Could you check a few things on this model? Use its own coordinates, in mm. Face numbers are marked on the shaded views. A direction names the side the tool comes from. Give positions to 0.01 mm unless a question says otherwise; leave off trailing zeros. Write each loop counter-clockwise with the first axis right and the second up, starting at its lowest first coordinate (ties: lowest second). Pieces come first, ordered by that corner, then holes. Notation, with made-up numbers: (-9.5, -5.75) -> (37.5, -5.75) arc R11 ccw to (37.5, 3.25) -> close; hole circle Ø8 at (74, 76.5). An arc over 180 degrees is marked (long way). Write item = value, one per line. Start each with the question number.
Autodesk Inventor part; units mm, degrees
ref_plane "XZ Plane" through (0, 0, 0) normal (0, 1, 0) x (-1, 0, 0)
ref_plane "XY Plane" through (0, 0, 0) normal (0, 0, 1) x (1, 0, 0)
sketch "Skizze1" plane through (0, 0, 0) normal (1, 0, 0) x (0, 1, 0)
  line L0 (15, -20) -> (5, -20)
  line L1 (5, -20) -> (5, -25)
  line L2 (5, -25) -> (15, -25)
  line L3 (15, -25) -> (15, -20)
  line L4 (5, -20) -> (0, -20)
  line L5 (0, -20) -> (0, -55)
  line L6 (0, -55) -> (5, -55)
  line L7 (5, -55) -> (5, -20)
  line L8 (0, -47) -> (-15, -47)
  line L9 (-15, -47) -> (-15, -42)
  line L10 (-15, -42) -> (0, -42)
  line L11 (0, -42) -> (0, -47)
  line L12 (0, -42) -> (-2, -42)
  line L13 (-2, -42) -> (-2, -37.5)
  line L14 (-2, -37.5) -> (0, -37.5)
  line L15 (0, -37.5) -> (0, -42)
  line L16 (-21, 0) -> (21, 0)
  line L17 (0, -66) -> (0, 11)
  point P0 (0, 0)
  point P1 (10, -25)
  point P2 (10, -20)
  point P3 (0, -44.5)
  point P4 (2.5, -55)
  point P5 (-7.5, -47)
  point P6 (0, -37.5)
  point P7 (-2, -42)
  point P8 (5, -25)
  dimension "d0" = 5
  dimension "d1" = 5
  dimension "d2" = 35
  dimension "d3" = 10
  dimension "d4" = 8
  dimension "d5" = 5
  dimension "d6" = 15
  dimension "d7" = 20
  dimension "d8" = 2
  dimension "d9" = 4.5
  dimension "d10" = 0
revolve "Umdrehung1" add sketch "Skizze1" angle 360 about axis through (0, -10, 0) along (0, 1, 0)
fillet "Rundung1" radius 3 1 edges at (0, 5, 25)
fillet "Rundung2" radius 2 1 edges at (0, -2, 42)
sketch "Skizze2" plane through (0, 5, 0) normal (0, 1, 0) x (1, 0, 0)
  line L0 (-77, 0) -> (77, 0)
  line L1 (0, 77) -> (0, -77)
  circle A0 centre (0, 0) radius 51
  circle A1 centre (0, 0) radius 55
  point P0 (0, -51)
  point P1 (44.1673, -25.5)
  point P2 (44.1673, 25.5)
  point P3 (0, 51)
  point P4 (-44.1673, 25.5)
  point P5 (-44.1673, -25.5)
  dimension "d14" = 4
  dimension "d17" = 360
hole "Bohrung1" at (0, 5, 51) at (44.1673, 5, 25.5) at (44.1673, 5, -25.5) at (0, 5, -51) at (-44.1673, 5, -25.5) at (-44.1673, 5, 25.5) direction (0, -1, 0) diameter 4.5 depth 11.8 tip angle 118
properties part number "Deckel Stempel"
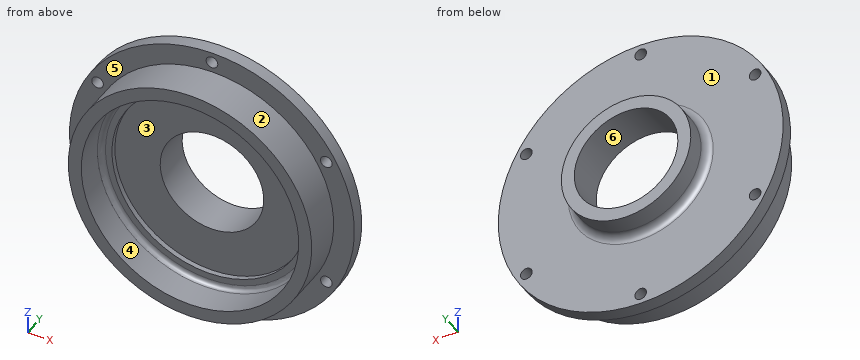
(1) Imagine slicing it at C-C (y = -13). Please give me the cut outline in (x, z), then the cut area to 3 significant figures.
(2) Imagine slicing it at D-D (z = 45.5). Please give me the cut outline in (x, y).
(3) We'd pull the mould along X, two halves only. Please class the marked faces 1, 2, 3 and 4: released by +X, released by -X, zero draft, split by the parting line, or undercut.
(4) On a 3-axis mill with a long thin cutter (end or side, diameter ignored), from which of +Z, -Z, +X, -X, +Y, -Y can I reach the whole of each face in a straight line? I mean the marked faces 5 and 6. Say none if no direction works.
(5) Imagine slicing it at A-A (z = 0). Please give me the cut outline in (x, y), then the cut area to 3 significant figures.
(6) If I drill on line 1 along X through (y, z) = (2.8, 25.5); line 2 along Z through (x, y) = (0, 11.75); line 3 along Y through (x, z) = (45, -30.5), over which ranges is the centre line in solid material (lowest first)? Write a range as from..to.
(7) Imagine slicing it at B-B (x = 0). State how many separate pieces and enclosed holes the cut face has, then the cut area to 3 significant figures.
(8) I'm going to push flat-ended pins straight in: pin 1 (2.5 mm diameter, centred on x = 0, z = -51, fed in from +Y); pin 2 (5 mm diameter, centred on x = 37, z = -6.5, fed in from -Y); pin 3 (6 mm diameter, centred on x = 24.5, z = 20.5, fed in from -Y); pin 4 (2 mm diameter, centred on x = -37, y = 3, fed in from -Z). Where does each tip first touch, or does it pass through?
Answers below:
q1.outline = circle Ø94 at (0, 0); hole circle Ø84 at (0, 0)
q1.area = 1,400 mm^2
q2.outline = (-30.9, 0) -> (-11.78, 0) -> (-11.78, -15) -> (11.78, -15) -> (11.78, 0) -> (30.9, 0) -> (30.9, 5) -> (-30.9, 5) -> close
q3.face_1 = zero draft
q3.face_2 = split by the parting line
q3.face_3 = undercut
q3.face_4 = undercut
q4.face_5 = -Y
q4.face_6 = +Y, -Y
q5.outline = (-55, 0) -> (-47, 0) -> (-47, -15) -> (-42, -15) -> (-42, -4) arc R2 cw to (-40, -2) -> (-37.5, -2) -> (-37.5, 0) -> (-20, 0) -> (-20, 15) -> (-25, 15) -> (-25, 8) arc R3 cw to (-28, 5) -> (-55, 5) -> close; (20, 0) -> (37.5, 0) -> (37.5, -2) -> (40, -2) arc R2 cw to (42, -4) -> (42, -15) -> (47, -15) -> (47, 0) -> (55, 0) -> (55, 5) -> (28, 5) arc R3 cw to (25, 8) -> (25, 15) -> (20, 15) -> close
q5.area = 624 mm^2
q6.line_1 = -48.73..-46.42, -41.92..41.92, 46.42..48.73
q6.line_2 = -25..-20, 20..25
q6.line_3 = 0..5
q7.separate_pieces = 4
q7.enclosed_holes = 0
q7.area = 579 mm^2
q8.pin_1 = through
q8.pin_2 = -2
q8.pin_3 = 0
q8.pin_4 = -41.58
